CAD build for the part. Positions are in the model's coordinates, mm. A direction names the side the tool comes from. Round coordinates to 2 decimals unless told otherwise and drop trailing zeros. Write each loop counter-clockwise with the first axis right and the second up, starting at its lowest first coordinate (ties: lowest second). Pieces come first, ordered by that corner, then holes. Notation, with made-up numbers: (82, -34) - (120, -34) arc R20 ccw to (120, -5) - close; hole circle Ø3 at (28.25, 75). An arc over 180 degrees is marked (long way). Use one line per item in the form item = value. Start each with the question number.
Item 1: Band-saw the part on C-C, the plane z = 0. List the corners of the cut face in (x, y), and give its area (3 significant figures).
Item 2: Band-saw the part on A-A, the plane y = -29.5. Give the number of separate pieces and of enclosed holes in the cut face, and give its area (3 significant figures).
Item 3: Drill centre lines: L1, parallel to Z at x = -38.5, y = -32; L2, parallel to X at y = -47, z = 17; L3, parallel to Z at x = 49, y = -43. Where is each one in solid material? Low to high.
Item 4: Band-saw the part on D-D, the plane x = -32.5. List the corners of the cut face in (y, z), and give its area (3 significant figures).
Item 5: Pull direction X, two halves, no side cores. Call faces 4 (the flat face through (-1, -25, 38.1)), 5 (the conical face through (38.9, -22.25, -16.79)), 6 (the flat face through (63.5, -25, 0)): +X half, -X half, draft (parallel to the pull), parting line (faces both ways), or undercut.
Item 6: Tool access for faces 1 (the cylindrical face through (-37.425, -46.28, 16.599)), 2 (the flat face through (-1, -44.45, 0)), 3 (the cylindrical face through (60.37, -40.58, 0.55)): list every direction of +Z, -Z, +X, -X, +Y, -Y with a clear straight run to the whole face (end or side of a thin tool).
Item 7: Pin check, flat tips, straight feed: pin 1 (7.5 mm diameter, centred on x = -39, z = 19, fed in from +Y); pin 2 (4 mm diameter, centred on x = 22.5, z = -2.5, fed in from +Y); pin 3 (3.5 mm diameter, centred on x = 38.68, z = -16.76, fed in from -Y); pin 4 (2 mm diameter, centred on x = 38.68, z = 16.76, fed in from -Y). Stop position of each tip, or through.
Item 8: Band-saw the part on B-B, the plane y = -7.5. List the corners of the cut face in (x, z) (3 decimals), and give its area (3 significant figures).
from build123d import *

# Parameters (mm, degrees)
SKETCH1_W                 = 127
SKETCH1_H                 = 76.2
BOSS_EXTRUDE1_DEPTH       = 50.8
FILLET1_R                 = 9.525
SHELL2_T                  = -6.35
SKETCH2_R                 = 3.175
BOSS_EXTRUDE2_DEPTH       = 44.45
MIRROR2_COPY_1_SKETCH_R   = 3.175
MIRROR2_COPY_1_DEPTH      = 44.45
F_6_40_TAPPED_HOLE1_D     = 2.8702
F_6_40_TAPPED_HOLE1_DEPTH = 12.7
F_6_40_TAPPED_HOLE1_TIP   = 0.862295074
SKETCH4_R                 = 4.7625
BOSS_EXTRUDE3_DEPTH       = 31.75
F_6_40_TAPPED_HOLE2_D     = 2.54
F_6_40_TAPPED_HOLE2_DEPTH = 8.9154
F_6_40_TAPPED_HOLE2_TIP   = 0.763092986
SKETCH7_R                 = 2.667
CUT_EXTRUDE1_DEPTH        = 12.7
SKETCH8_R                 = 2.54
CUT_EXTRUDE2_DEPTH        = 13.97
F_6_40_TAPPED_HOLE3_D     = 2.54
F_6_40_TAPPED_HOLE3_DEPTH = 8.9154
F_6_40_TAPPED_HOLE3_TIP   = 0.763092986


with BuildPart() as part:
    # Sketch1 → Boss-Extrude1 (new body)
    with BuildSketch(Plane(origin=(0, 0, 0), x_dir=(1, 0, 0), z_dir=(0, 1, 0))):
        Rectangle(SKETCH1_W, SKETCH1_H)
    extrude(amount=-BOSS_EXTRUDE1_DEPTH)

    # Fillet1
    fillet1_edges = [part.edges().sort_by_distance(p)[0] for p in [
        (63.5, -25.4, 38.1),
        (-63.5, -25.4, 38.1),
        (-63.5, -25.4, -38.1),
        (63.5, -25.4, -38.1),
    ]]
    fillet(fillet1_edges, radius=FILLET1_R)

    # Shell2
    shell2_openings = [part.faces().sort_by_distance(p)[0] for p in [
        (0, 0, 0),
    ]]
    offset(amount=SHELL2_T, openings=shell2_openings, kind=Kind.INTERSECTION)

    # Sketch2 → Boss-Extrude2 (add)
    with BuildSketch(Plane(origin=(0, -44.45, 0), x_dir=(1, 0, 0), z_dir=(0, 1, 0))):
        with Locations((-53.975, 28.575)):
            Circle(SKETCH2_R)
    boss_extrude2 = extrude(amount=BOSS_EXTRUDE2_DEPTH)

    # Mirror1: Boss-Extrude2 across plane
    add(boss_extrude2.mirror(Plane(origin=(0, 0, 0), x_dir=(0, 0, 1), z_dir=(1, 0, 0))))

    # Mirror2: Boss-Extrude2 across plane
    add(boss_extrude2.mirror(Plane.XY))

    # Mirror2 copy 1 sketch → Mirror2 copy 1 (add)
    with BuildSketch(Plane(origin=(0, -44.45, 0), x_dir=(-1, 0, 0), z_dir=(0, 1, 0))):
        with Locations((-53.975, 28.575)):
            Circle(MIRROR2_COPY_1_SKETCH_R)
    extrude(amount=MIRROR2_COPY_1_DEPTH)

    # #6-40 Tapped Hole1
    with Locations(Plane(origin=(-53.975, 0, -28.575), x_dir=(0, 0, 1), z_dir=(0, 1, 0))):
        with Locations((0, 0), (57.15, 0), (57.15, 107.95), (0, 107.95)):
            Hole(F_6_40_TAPPED_HOLE1_D / 2, depth=F_6_40_TAPPED_HOLE1_DEPTH)
            with Locations((0, 0, -(F_6_40_TAPPED_HOLE1_DEPTH + F_6_40_TAPPED_HOLE1_TIP / 2))):  # 118° drill point
                Cone(0, F_6_40_TAPPED_HOLE1_D / 2, F_6_40_TAPPED_HOLE1_TIP, mode=Mode.SUBTRACT)

    # Sketch4 → Boss-Extrude3 (add)
    with BuildSketch(Plane(origin=(0, -44.45, 0), x_dir=(1, 0, 0), z_dir=(0, 1, 0))):
        with Locations(Location((-38.6842, 16.764, 0), (0, 0, 90))):
            Circle(SKETCH4_R)
        with Locations(Location((38.6842, 16.764, 0), (0, 0, 90))):
            Circle(SKETCH4_R)
        with Locations(Location((-38.6842, -16.764, 0), (0, 0, 90))):
            Circle(SKETCH4_R)
        with Locations(Location((38.6842, -16.764, 0), (0, 0, 90))):
            Circle(SKETCH4_R)
    extrude(amount=BOSS_EXTRUDE3_DEPTH)

    # #6-40 Tapped Hole2
    with Locations(Plane(origin=(-38.6842, -12.7, -16.764), x_dir=(0, 0, 1), z_dir=(0, 1, 0))):
        with Locations((0, 0), (0, 77.3684), (33.528, 0), (33.528, 77.3684)):
            Hole(F_6_40_TAPPED_HOLE2_D / 2, depth=F_6_40_TAPPED_HOLE2_DEPTH)
            with Locations((0, 0, -(F_6_40_TAPPED_HOLE2_DEPTH + F_6_40_TAPPED_HOLE2_TIP / 2))):  # 118° drill point
                Cone(0, F_6_40_TAPPED_HOLE2_D / 2, F_6_40_TAPPED_HOLE2_TIP, mode=Mode.SUBTRACT)

    # Sketch7 → Cut-Extrude1 (cut)
    with BuildSketch(Plane.ZY.offset(63.5)):
        with Locations((0, -38.1)):
            Circle(SKETCH7_R)
    extrude(amount=-CUT_EXTRUDE1_DEPTH, mode=Mode.SUBTRACT)

    # Sketch8 → Cut-Extrude2 (cut)
    with BuildSketch(Plane(origin=(63.5, 0, 0), x_dir=(0, 0, -1), z_dir=(1, 0, 0))):
        with Locations((0, -38.1)):
            Circle(SKETCH8_R)
    extrude(amount=-CUT_EXTRUDE2_DEPTH, mode=Mode.SUBTRACT)

    # #6-40 Tapped Hole3
    with Locations(Plane(origin=(-38.6842, -50.8, -16.764), x_dir=(0, 0, -1), z_dir=(0, -1, 0))):
        with Locations((0, 0), (-33.528, 0), (-33.528, 77.3684), (0, 77.3684)):
            Hole(F_6_40_TAPPED_HOLE3_D / 2, depth=F_6_40_TAPPED_HOLE3_DEPTH)
            with Locations((0, 0, -(F_6_40_TAPPED_HOLE3_DEPTH + F_6_40_TAPPED_HOLE3_TIP / 2))):  # 118° drill point
                Cone(0, F_6_40_TAPPED_HOLE3_D / 2, F_6_40_TAPPED_HOLE3_TIP, mode=Mode.SUBTRACT)


solid = part.part
Determined:
q1.outline = (-63.5, -50.8) - (63.5, -50.8) - (63.5, -40.64) - (57.15, -40.64) - (57.15, -44.45) - (-57.15, -44.45) - (-57.15, -40.77) - (-63.5, -40.77) - close; (-63.5, -35.43) - (-57.15, -35.43) - (-57.15, 0) - (-63.5, 0) - close; (57.15, -35.56) - (63.5, -35.56) - (63.5, 0) - (57.15, 0) - close
q1.area = 1,300 mm²
q2.separate_pieces = 5
q2.enclosed_holes = 1
q2.area = 2,760 mm²
q3.L1 = -38.1 to -31.75, -21.52 to -12.01, 12.01 to 21.52, 31.75 to 38.1
q3.L2 = -63.5 to -39.93, -37.44 to 37.44, 39.93 to 63.5
q3.L3 = -38.1 to -31.75, 31.75 to 38.1
q4.outline = (-50.8, -38.1) - (0, -38.1) - (0, -31.75) - (-44.45, -31.75) - (-44.45, 31.75) - (0, 31.75) - (0, 38.1) - (-50.8, 38.1) - close
q4.area = 1,050 mm²
q5.face_4 = draft
q5.face_5 = undercut
q5.face_6 = +X half
q6.face_1 = -Y
q6.face_2 = +Y
q6.face_3 = +X, -X
q7.pin_1 = -12.7
q7.pin_2 = -44.45
q7.pin_3 = -50.8
q7.pin_4 = -41.73
q8.outline = (-63.5, -28.575) arc R9.525 ccw to (-53.975, -38.1) - (53.975, -38.1) arc R9.525 ccw to (63.5, -28.575) - (63.5, 28.575) arc R9.525 ccw to (53.975, 38.1) - (-53.975, 38.1) arc R9.525 ccw to (-63.5, 28.575) - close; hole (-57.15, -28.575) arc R3.175 cw (long way) to (-53.975, -31.75) - (53.975, -31.75) arc R3.175 cw (long way) to (57.15, -28.575) - (57.15, 28.575) arc R3.175 cw (long way) to (53.975, 31.75) - (-53.975, 31.75) arc R3.175 cw (long way) to (-57.15, 28.575) - close; hole circle Ø2.87 at (-53.975, -28.575); hole circle Ø2.87 at (-53.975, 28.575); hole circle Ø2.87 at (53.975, -28.575); hole circle Ø2.87 at (53.975, 28.575)
q8.area = 2,450 mm²
